Could you check a few things on this model? Use its own coordinates, in mm. Coordinates: 2 decimals unless noted, no trailing zeros. Write each loop counter-clockwise with the first axis right and the second up, starting at its lowest first coordinate (ties: lowest second). Pieces come first, ordered by that corner, then holes.
```python
from build123d import *

# Parameters (mm, degrees)
F0_W     = 44.45
F0_H     = 57.15
F1_DEPTH = 15.24
F2_SIZE  = 11.43
F3_R     = 10.795
F4_DEPTH = 25.4
F6_DEPTH = 76.2


with BuildPart() as f1:
    # F0 (on Top) → F1 (new body)
    with BuildSketch(Plane.XY):
        with Locations((22.225, 28.575)):
            Rectangle(F0_W, F0_H)
    extrude(amount=F1_DEPTH)

    # F2
    f2_edges = [f1.edges().sort_by_distance(p)[0] for p in [
        (0, 0, 7.62),
        (44.45, 0, 7.62),
    ]]
    chamfer(f2_edges, length=F2_SIZE)

    # F3 (on face) → F4 (cut)
    with BuildSketch(Plane.XY.offset(15.24)):
        with Locations((22.225, 16.51)):
            Circle(F3_R)
    extrude(amount=-F4_DEPTH, mode=Mode.SUBTRACT)

    # F5 (on face) → F6 (cut)
    with BuildSketch(Plane.YZ.offset(44.45)):
        with BuildLine():
            Line((52.07, 15.24), (31.75, 15.24))
            ThreePointArc((31.75, 15.24), (41.91, 5.08), (52.07, 15.24))
        make_face()
    extrude(amount=-F6_DEPTH, mode=Mode.SUBTRACT)


solid = f1.part
```
1. I want a section at D-D on x = 5.5. Please give me the cut outline in (y, z), plus the area to 3 significant figures.
Verdict:
outline: (5.93, 0) - (57.15, 0) - (57.15, 15.24) - (52.07, 15.24) arc R10.16 cw to (31.75, 15.24) - (5.93, 15.24) - close
area: 618 mm2
2. For pin 1 (2 mm diameter, centred on y = 9, z = 8, fed in from -X), with a flat end and sliding along its axis, tell me the tip position at first contact or that it passes through.
Verdict:
pin 1: stops at x = 1.43
3. I want a section at A-A on y = 16.51. Please give me the cut outline in (x, z).
Verdict:
outline: (0, 0) - (11.43, 0) - (11.43, 15.24) - (0, 15.24) - close; (33.02, 0) - (44.45, 0) - (44.45, 15.24) - (33.02, 15.24) - close
4. I want a section at C-C on x = 32. Please give me the cut outline in (y, z).
Verdict:
outline: (0, 0) - (11.93, 0) - (11.93, 15.24) - (0, 15.24) - close; (21.09, 0) - (57.15, 0) - (57.15, 15.24) - (52.07, 15.24) arc R10.16 cw to (31.75, 15.24) - (21.09, 15.24) - close
5. Please list where these lines run through material, in increasing order: line 1 along Y through (x, z) = (31.5, 7.5); line 2 along Y through (x, z) = (23, 13); line 3 along Y through (x, z) = (19, 2).
Verdict:
line 1: y = 0 to 10.99, 22.03 to 35.33, 48.49 to 57.15
line 2: y = 0 to 5.74, 27.28 to 32, 51.82 to 57.15
line 3: y = 0 to 6.21, 26.81 to 57.15
6. I want a section at B-B on z = 9. Please give me the cut outline in (x, y) (3 decimals).
Verdict:
outline: (0, 11.43) - (11.43, 0) - (33.02, 0) - (44.45, 11.43) - (44.45, 33.892) - (0, 33.892) - close; (0, 49.928) - (44.45, 49.928) - (44.45, 57.15) - (0, 57.15) - close; hole circle Ø21.59 at (22.225, 16.51)
7. If we mould it in two halves opening along Y, with no side actions, what happens to faces 1 (the face through (11.44, 16.98, 7.73)), 2 (the face through (5.8, 5.63, 7.51)), 3 (the face through (27, 27, 15.24))? For each: pulls with the +Y half, pulls with the -Y half, needs draft (parallel to the pull), parting line crosses it, or undercut.
Verdict:
face 1: undercut
face 2: pulls with the -Y half
face 3: needs draft
